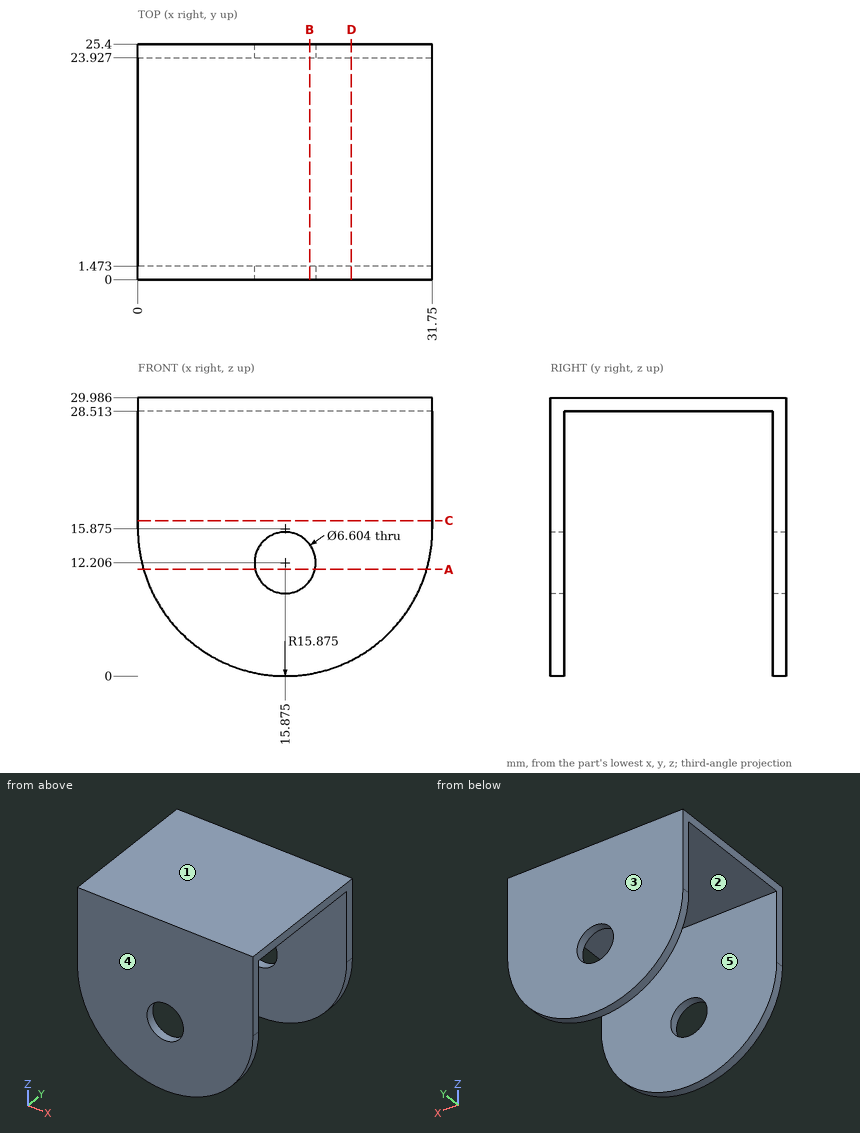
Job drawing, mm, ordinate dimensions from the low corner. One solid piece. A direction names the side the tool comes from. Coordinates: 2 decimals unless noted, no trailing zeros. Order: outer loops, then holes, each group sorted by start corner. A loop starts at its lowest first (then second) coordinate and runs counter-clockwise, first axis right, second up. Notation, with made-up numbers: (-30, 78) - (4, 78) arc R10 cw to (4, 95) - close; hole circle Ø2 at (16, -4.75). An arc over 180 degrees is marked (long way). Return JSON: item names as keys, results as strings. Group by question number.
1) Saw through at D-D, the plane x = 23. Write the cut outline in (y, z).
2) Mould opens along Y. For the marked faces 3, 4 and 5 say: released by +Y, released by -Y, zero draft, split by the parting line, or undercut.
3) Saw through at C-C, the plane z = 16.75. Write the cut outline in (x, y).
4) Saw through at A-A, the plane z = 11.5. Write the cut outline in (x, y) (1 decimal).
5) Probe line 1 (Y direction, x = 10, z = 27.5); line 2 (Z direction, x = 25, y = 2.25). List the from-to ranges inside material, lowest first. Write a range as from..to.
6) Tool access for the marked faces 1 and 2: list every direction of +Z, -Z, +X, -X, +Y, -Y with a clear straight run to the whole face (end or side of a thin tool).
7) Saw through at B-B, the plane x = 18.5. Write the cut outline in (y, z), plus the area to 3 significant figures.
8) Flat gauge pins, fed straight in: P1, Ø6.5, axis at x = 12.5, y = 14, coming from the -Z side; P2, Ø8, axis at y = 12, z = 22, coming from the -X side. Where does each tip first touch, or does it go through?
Values found:
{
 "1": {"outline": "(0, 1.69) - (1.47, 1.69) - (1.47, 28.51) - (23.93, 28.51) - (23.93, 1.69) - (25.4, 1.69) - (25.4, 29.99) - (0, 29.99) - close"},
 "2": {"face 3": "released by +Y", "face 4": "released by -Y", "face 5": "undercut"},
 "3": {"outline": "(0, 0) - (31.75, 0) - (31.75, 1.47) - (0, 1.47) - close; (0, 23.93) - (31.75, 23.93) - (31.75, 25.4) - (0, 25.4) - close"},
 "4": {"outline": "(0.6, 0) - (12.6, 0) - (12.6, 1.5) - (0.6, 1.5) - close; (0.6, 23.9) - (12.6, 23.9) - (12.6, 25.4) - (0.6, 25.4) - close; (19.1, 0) - (31.1, 0) - (31.1, 1.5) - (19.1, 1.5) - close; (19.1, 23.9) - (31.1, 23.9) - (31.1, 25.4) - (19.1, 25.4) - close"},
 "5": {"line 1": "y = 0..1.47, 23.93..25.4", "line 2": "z = 28.51..29.99"},
 "6": {"face 1": "+Z, +X, -X, +Y, -Y", "face 2": "-Z, +X, -X"},
 "7": {"outline": "(0, 0.22) - (1.47, 0.22) - (1.47, 10.2) - (0, 10.2) - close; (0, 14.21) - (1.47, 14.21) - (1.47, 28.51) - (23.93, 28.51) - (23.93, 14.21) - (25.4, 14.21) - (25.4, 29.99) - (0, 29.99) - close; (23.93, 0.22) - (25.4, 0.22) - (25.4, 10.2) - (23.93, 10.2) - close", "area": "109 mm²"},
 "8": {"P1": "stops at z = 28.51", "P2": "passes through"}
}
